Can you work these out from the drawing? Everything is in mm from the part's minimum corner. Give positions to 0.01 mm unless a question says otherwise; leave off trailing zeros. Loops run counter-clockwise (first coordinate to the right, second up) from the corner with the lowest first, then second, coordinate; pieces in that order, holes last. Notation, with made-up numbers: M 68.25,-32 L 125.25,-32 A22 cw 125.25,-14 Z; hole C 88,19.25 d1. An arc over 180 degrees is marked long. Use CSV: the item, a comma, the result in double quotes.
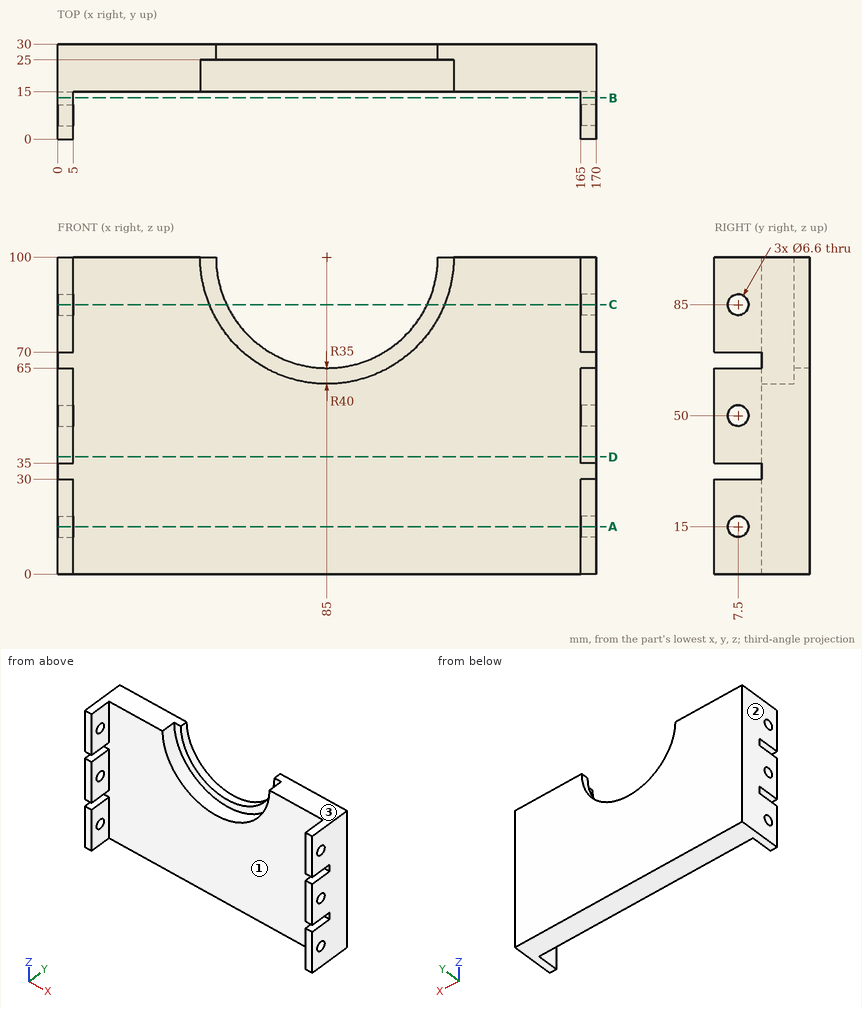
Q1. Please list where these lines run through material, in increasing order: L1, parallel to Z at x = 2.3, y = 7.5; L2, parallel to X at y = 14.25, z = 9; L3, parallel to Y at x = 2, z = 50. Write a range as from..to.
Model answer:
L1,"0..11.7, 18.3..30, 35..46.7, 53.3..65, 70..81.7, 88.3..100"
L2,"0..5, 165..170"
L3,"0..4.2, 10.8..30"
Q2. I'm going to push flat-ended pins straight in: P1, Ø8.5, axis at y = 7.5, z = 50, coming from the -X side; P2, Ø12, axis at x = 104, z = 70.5, coming from the -Y side. Where does each tip first touch, or does it pass through?
Model answer:
P1,"x = 0"
P2,"y = 15"
Q3. I want a section at C-C, the plane z = 85. Please give me the cut outline in (x, y), then the cut area to 3 significant figures.
Model answer:
outline,"M 0,0 L 5,0 L 5,4.2 L 0,4.2 Z; M 0,10.8 L 5,10.8 L 5,15 L 47.92,15 L 47.92,25 L 53.38,25 L 53.38,30 L 0,30 Z; M 116.62,25 L 122.08,25 L 122.08,15 L 165,15 L 165,10.8 L 170,10.8 L 170,30 L 116.62,30 Z; M 165,0 L 170,0 L 170,4.2 L 165,4.2 Z"
area,"1,580 mm2"
Q4. I want a section at D-D, the plane z = 37. Please give me the cut outline in (x, y).
Model answer:
outline,"M 0,0 L 5,0 L 5,15 L 165,15 L 165,0 L 170,0 L 170,30 L 0,30 Z"
Q5. If we mould it in two halves opening along X, with no side actions, what happens to the marked faces 1, 2 and 3? For each: released by +X, released by -X, zero draft, split by the parting line, or undercut.
Model answer:
face 1,"undercut"
face 2,"released by -X"
face 3,"zero draft"
Q6. I want a section at A-A, the plane z = 15. Please give me the cut outline in (x, y), then the cut area to 3 significant figures.
Model answer:
outline,"M 0,0 L 5,0 L 5,4.2 L 0,4.2 Z; M 0,10.8 L 5,10.8 L 5,15 L 165,15 L 165,10.8 L 170,10.8 L 170,30 L 0,30 Z; M 165,0 L 170,0 L 170,4.2 L 165,4.2 Z"
area,"2,630 mm2"
Q7. I want a section at B-B, the plane y = 13. Please give me the cut outline in (x, z), then the cut area to 3 significant figures.
Model answer:
outline,"M 0,0 L 5,0 L 5,30 L 0,30 Z; M 0,35 L 5,35 L 5,65 L 0,65 Z; M 0,70 L 5,70 L 5,100 L 0,100 Z; M 165,0 L 170,0 L 170,30 L 165,30 Z; M 165,35 L 170,35 L 170,65 L 165,65 Z; M 165,70 L 170,70 L 170,100 L 165,100 Z"
area,"900 mm2"
